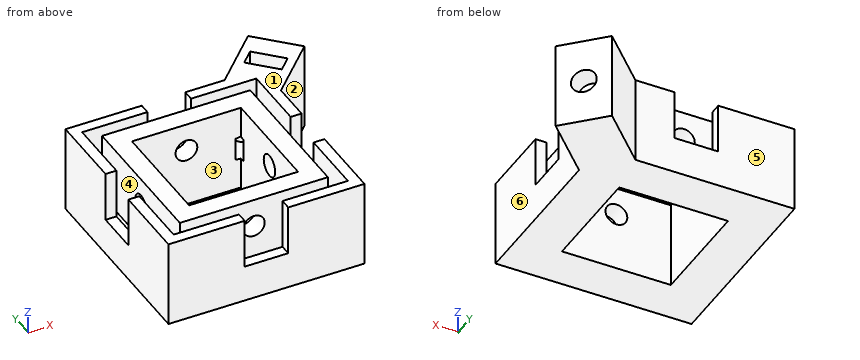
from build123d import *

# Parameters (mm, degrees)
F0_W      = 25
F0_H      = 25
F1_DEPTH  = 5
F2_W      = 34
F2_H      = 34
F2_W_2    = 25
F2_H_2    = 25
F3_DEPTH  = 15
F4_W      = 40
F4_H      = 40
F5_DEPTH  = 15
F6_W      = 10
F6_H      = 2.5
F6_W_2    = 2.5
F6_H_2    = 10
F7_DEPTH  = 11.5
F8_R      = 2.75
F9_DEPTH  = 25
F11_DEPTH = 15
F12_R     = 2.5
F13_DEPTH = 45
F14_R     = 2.5
F15_DEPTH = 45


with BuildPart() as f1:
    # F0 (on Top) → F1 (new body)
    with BuildSketch(Plane.XY):
        Polygon((22.5, 14.0147186258), (22.5, 22.5), (14.0147186258, 22.5), (-22.5, 22.5), (-22.5, -22.5), (22.5, -22.5), align=None)
        Rectangle(F0_W, F0_H, mode=Mode.SUBTRACT)
        Polygon((14.0147186258, 22.5), (22.5, 22.5), (22.5, 14.0147186258), (33.813708499, 25.3284271247), (25.3284271247, 33.813708499), align=None)
    extrude(amount=F1_DEPTH)

    # F2 (on face) → F3 (join)
    with BuildSketch(Plane.XY.offset(5)):
        Rectangle(F2_W, F2_H)
        Rectangle(F2_W_2, F2_H_2, mode=Mode.SUBTRACT)
    extrude(amount=F3_DEPTH)

    # F4 (on face) → F5 (join)
    with BuildSketch(Plane.XY.offset(5)):
        Polygon((25.3284271247, 33.813708499), (14.0147186258, 22.5), (-22.5, 22.5), (-22.5, -22.5), (22.5, -22.5), (22.5, 14.0147186258), (33.813708499, 25.3284271247), align=None)
        Rectangle(F4_W, F4_H, mode=Mode.SUBTRACT)
    extrude(amount=F5_DEPTH)

    # F6 (on face) → F7 (cut)
    with BuildSketch(Plane.XY.offset(20)):
        with Locations((0, 21.25)):
            Rectangle(F6_W, F6_H)
        with Locations((-21.25, 0)):
            Rectangle(F6_W_2, F6_H_2)
        with Locations((21.25, 0)):
            Rectangle(F6_W_2, F6_H_2)
        with Locations((0, -21.25)):
            Rectangle(F6_W, F6_H)
    extrude(amount=-F7_DEPTH, mode=Mode.SUBTRACT)

    # F8 (on face) → F9 (cut)
    with BuildSketch(Plane(origin=(29.5710678119, 29.5710678119, 0), x_dir=(-0.7071067812, 0.7071067812, 0), z_dir=(0.7071067812, 0.7071067812, 0))):
        with Locations((0, 10)):
            Circle(F8_R)
    extrude(amount=-F9_DEPTH, mode=Mode.SUBTRACT)

    # F10 (on face) → F11 (cut)
    with BuildSketch(Plane.XY.offset(20)):
        Polygon((28.8639610307, 23.2071067812), (23.2071067812, 28.8639610307), (20.3786796564, 26.0355339059), (26.0355339059, 20.3786796564), align=None)
    extrude(amount=-F11_DEPTH, mode=Mode.SUBTRACT)

    # F12 (on face) → F13 (cut)
    with BuildSketch(Plane(origin=(0, 17, 0), x_dir=(-1, 0, 0), z_dir=(0, 1, 0))):
        with Locations((0, 13.5)):
            Circle(F12_R)
    extrude(amount=-F13_DEPTH, mode=Mode.SUBTRACT)

    # F14 (on face) → F15 (cut)
    with BuildSketch(Plane.YZ.offset(17)):
        with Locations((0, 13.5)):
            Circle(F14_R)
    extrude(amount=-F15_DEPTH, mode=Mode.SUBTRACT)


solid = f1.part
Part model, mm, in its own coordinate system. Face numbers are marked on the shaded views. A direction names the side the tool comes from. Give positions to 0.01 mm unless a question says otherwise; leave off trailing zeros. Loops run counter-clockwise (first coordinate to the right, second up) from the corner with the lowest first, then second, coordinate; pieces in that order, holes last. Notation, with made-up numbers: M -6.5,35.5 L 26.5,35.5 A3 cw 26.5,40.5 Z; hole C 14.25,4 d8. An arc over 180 degrees is marked long. Put each result on its own line as item: value. Start each with the question number.
1) Saw through at C-C (y = -8). List the corners of the cut face in (x, z).
2) Probe probe 1 along Y at (x, z) = (-9, 10.5); probe 2 along Z at (x, y) = (0, 13.95); probe 3 along Y at (x, z) = (2.5, 13). List the from-to ranges inside material, lowest first.
3) Pull direction Y, two halves, no side cores. Call the marked faces 1, 2 and 3: +Y half, -Y half, draft (parallel to the pull), parting line (faces both ways), or undercut.
4) Saw through at A-A (x = -1.5). List the corners of the cut face in (y, z), then the cut area to 4 significant figures.
5) Saw through at B-B (y = 0). List the corners of the cut face in (x, z).
6) Saw through at D-D (z = 13.5). State how many separate pieces and enclosed holes the cut face has, then the cut area to 3 significant figures.
7) 3-axis set-ups, long thin cutter, end or side, ignore diameter. For the marked faces 4, 5 and 6: which of +Z, -Z, +X, -X, +Y, -Y reach the whole face in a straight line?
8) Flat gauge pins, fed straight in: pin 1 (3 mm diameter, centred on y = -21.5, z = 13, fed in from +X); pin 2 (4.5 mm diameter, centred on x = 0, z = 11.5, fed in from +Y); pin 3 (2 mm diameter, centred on x = -21, y = 1, fed in from +Z). Where does each tip first touch, or does it go through?
Numbers:
1. outline: M -22.5,0 L -12.5,0 L -12.5,20 L -17,20 L -17,5 L -20,5 L -20,20 L -22.5,20 Z; M 12.5,0 L 22.5,0 L 22.5,20 L 20,20 L 20,5 L 17,5 L 17,20 L 12.5,20 Z
2. probe 1: -22.5 to -20, -17 to -12.5, 12.5 to 17, 20 to 22.5
2. probe 2: 0 to 11, 16 to 20
2. probe 3: -17 to -12.5, 12.5 to 17
3. face 1: draft
3. face 2: -Y half
3. face 3: undercut
4. outline: M -22.5,0 L -12.5,0 L -12.5,11.5 L -17,11.5 L -17,5 L -20,5 L -20,8.5 L -22.5,8.5 Z; M -17,15.5 L -12.5,15.5 L -12.5,20 L -17,20 Z; M 12.5,0 L 22.5,0 L 22.5,8.5 L 20,8.5 L 20,5 L 17,5 L 17,11.5 L 12.5,11.5 Z; M 12.5,15.5 L 17,15.5 L 17,20 L 12.5,20 Z
4. area: 216.5 mm^2
5. outline: M -22.5,0 L -12.5,0 L -12.5,11 L -17,11 L -17,5 L -20,5 L -20,8.5 L -22.5,8.5 Z; M -17,16 L -12.5,16 L -12.5,20 L -17,20 Z; M 12.5,0 L 22.5,0 L 22.5,8.5 L 20,8.5 L 20,5 L 17,5 L 17,11 L 12.5,11 Z; M 12.5,16 L 17,16 L 17,20 L 12.5,20 Z
6. separate pieces: 8
6. enclosed holes: 1
6. area: 890 mm^2
7. face 4: +Z
7. face 5: +Z, -Z, -X, +Y
7. face 6: +Z, -Z, +X, -Y
8. pin 1: x = 22.5
8. pin 2: y = 17
8. pin 3: z = 8.5
